The figure shows three views and two pictorial views of one solid part (mm, origin at its lowest corner). Answer the questions. A direction names the side the tool comes from. Coordinates: 2 decimals unless noted, no trailing zeros. Loops run counter-clockwise (first coordinate to the right, second up) from the corner with the lowest first, then second, coordinate; pieces in that order, holes last. Notation, with made-up numbers: (-22, -7.5) -> (-14, -7.5) arc R16 ccw to (-14, -2.5) -> close; hole circle Ø10 at (78, 82). An arc over 180 degrees is marked (long way). Answer as a JSON object with one key per item and string values. Group by question number.
1) Section B-B, the plane z = 22.25 is taken. Give the vertices of the cut face in (x, y), plus the area to 3 significant figures.
2) Flat-ended cylindrical pins translate along their axes: P1, Ø6, axis at x = 35.5, y = 3.5, coming from the +Z side (1 decimal); P2, Ø2, axis at x = 29, z = 10, coming from the -Y side; P3, Ø6, axis at x = 32.5, y = 5, coming from the -Z side; P4, Ø5, axis at x = 22.25, z = 4.8, coming from the +Y side. Find the tip coordinate at first contact, or state that the pin passes through.
3) Section C-C, the plane y = 17 is taken. Give the vertices of the cut face in (x, z), plus the area to 4 significant figures.
4) Section D-D, the plane x = 36 is taken. Give the vertices of the cut face in (y, z).
5) Consider probe 1 along Z at (x, y) = (20, 6.5) (1 decimal); probe 2 along Y at (x, z) = (9.5, 13); probe 3 along Z at (x, y) = (21.5, 8) (1 decimal). Determine where each line is inside the solid, lowest interval first. Write a range as [from, to].
6) Determine the mould class of the marked faces 1, 2 and 3 for opening direction X: released by +X, released by -X, zero draft, split by the parting line, or undercut.
7) Which of the six approach directions +Z, -Z, +X, -X, +Y, -Y give full straight-line access (tool end or side, diameter ignored) to the marked faces 4, 5 and 6?
8) Section A-A, the plane x = 22.25 is taken. Give the vertices of the cut face in (y, z).
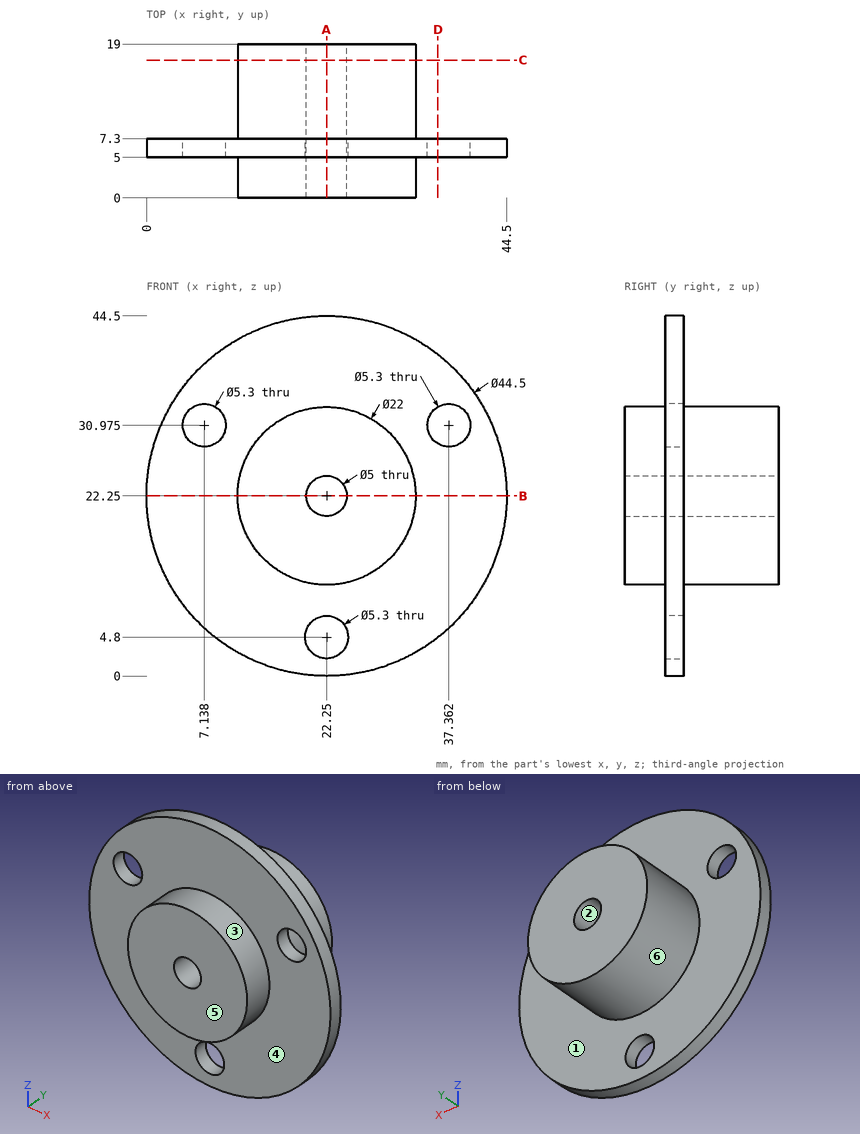
Determined:
{
 "1": {"outline": "(0, 5) -> (11.25, 5) -> (11.25, 0) -> (19.75, 0) -> (19.75, 19) -> (11.25, 19) -> (11.25, 7.3) -> (0, 7.3) -> close; (24.75, 0) -> (33.25, 0) -> (33.25, 5) -> (44.5, 5) -> (44.5, 7.3) -> (33.25, 7.3) -> (33.25, 19) -> (24.75, 19) -> close", "area": "375 mm²"},
 "2": {"P1": "z = 41.8", "P2": "y = 5", "P3": "z = 1.21", "P4": "through"},
 "3": {"outline": "circle Ø22 at (22.25, 22.25); hole circle Ø5 at (22.25, 22.25)", "area": "360.5 mm²"},
 "4": {"outline": "(5, 4.76) -> (7.3, 4.76) -> (7.3, 28.7) -> (5, 28.7) -> close; (5, 33.25) -> (7.3, 33.25) -> (7.3, 39.74) -> (5, 39.74) -> close"},
 "5": {"probe 1": "[0.1, 3.4], [6.2, 21.2], [23.3, 44.4]", "probe 2": "[5, 7.3]", "probe 3": "[11.3, 19.9], [24.6, 33.2]"},
 "6": {"face 1": "zero draft", "face 2": "undercut", "face 3": "split by the parting line"},
 "7": {"face 4": "-Y", "face 5": "+Z, -Z, +X, -X, -Y", "face 6": "+Y"},
 "8": {"outline": "(0, 11.25) -> (5, 11.25) -> (5, 7.45) -> (7.3, 7.45) -> (7.3, 11.25) -> (19, 11.25) -> (19, 19.75) -> (0, 19.75) -> close; (0, 24.75) -> (19, 24.75) -> (19, 33.25) -> (7.3, 33.25) -> (7.3, 44.5) -> (5, 44.5) -> (5, 33.25) -> (0, 33.25) -> close; (5, 0) -> (7.3, 0) -> (7.3, 2.15) -> (5, 2.15) -> close"}
}
